Autodesk Inventor part; units mm, degrees
ref_plane "YZ Plane" through (0, 0, 0) normal (1, 0, 0) x (0, 1, 0)
ref_plane "XZ Plane" through (0, 0, 0) normal (0, 1, 0) x (-1, 0, 0)
ref_plane "XY Plane" through (0, 0, 0) normal (0, 0, 1) x (1, 0, 0)
sketch "Esboço1" plane through (0, 0, 0) normal (1, 0, 0) x (0, 1, 0)
  line L0 (-504, 129) -> (504, 129)
  line L1 (504, 129) -> (504, -129)
  line L2 (504, -129) -> (-504, -129)
  line L3 (-504, -129) -> (-504, 129)
  line L4 (-504, 129) -> (504, -129) construction
  line L5 (504, 129) -> (-504, -129) construction
  point P0 (0, 0)
  dimension "d0" = 1008
  dimension "d1" = 258
extrude "Extrusão1" add sketch "Esboço1" along normal mid plane 4
sketch "Esboço2" plane through (2, 0, 0) normal (1, 0, 0) x (0, 0, -1)
  line L0 (-133, 378) -> (-125, 378)
  line L1 (-125, 378) -> (-125, 126)
  line L2 (-125, 126) -> (-133, 126)
  line L3 (-133, 126) -> (-133, 378)
  line L4 (-129, 504) -> (-129, -504)
  line L5 (-133, 378) -> (-125, 126) construction
  line L6 (-125, 378) -> (-133, 126) construction
  line L7 (129, 504) -> (-129, 504)
  line L8 (-133, -126) -> (-125, -126)
  line L9 (-125, -126) -> (-125, -378)
  line L10 (-125, -378) -> (-133, -378)
  line L11 (-133, -378) -> (-133, -126)
  line L12 (-133, -126) -> (-125, -378) construction
  line L13 (-125, -126) -> (-133, -378) construction
  line L14 (-129, -504) -> (129, -504)
  line L15 (125, 378) -> (133, 378)
  line L16 (133, 378) -> (133, 126)
  line L17 (133, 126) -> (125, 126)
  line L18 (125, 126) -> (125, 378)
  line L19 (129, -504) -> (129, 504)
  line L20 (125, 378) -> (133, 126) construction
  line L21 (133, 378) -> (125, 126) construction
  line L22 (125, -126) -> (133, -126)
  line L23 (133, -126) -> (133, -378)
  line L24 (133, -378) -> (125, -378)
  line L25 (125, -378) -> (125, -126)
  line L26 (125, -126) -> (133, -378) construction
  line L27 (133, -126) -> (125, -378) construction
  point P0 (0, 0)
  point P1 (-129, 252)
  point P2 (-129, -252)
  point P3 (129, 252)
  point P4 (129, -252)
  dimension "d4" = 8
  dimension "d5" = 252
  dimension "d6" = 126
  dimension "d7" = 8
  dimension "d8" = 252
  dimension "d9" = 252
  dimension "d10" = 126
  dimension "d11" = 126
  dimension "d12" = 252
  dimension "d13" = 8
  dimension "d14" = 252
  dimension "d15" = 8
  dimension "d16" = 252
  dimension "d17" = 126
extrude "Extrusão2" cut sketch "Esboço2" along normal through all both and the other way through all contours L0 L4 L2 L3 | L0 L1 L2 L4 | L8 L9 L10 L4 | L4 L10 L11 L8 | L19 L17 L18 L15 | L15 L16 L17 L19 | L22 L23 L24 L19 | L19 L24 L25 L22
sketch "Esboço3" plane through (2, 0, 0) normal (1, 0, 0) x (0, 0, -1)
  line L0 (-41.5, 500) -> (41.5, 500)
  line L1 (41.5, 500) -> (41.5, 508)
  line L2 (41.5, 508) -> (-41.5, 508)
  line L3 (-41.5, 508) -> (-41.5, 500)
  line L4 (129, 504) -> (-129, 504)
  line L5 (-41.5, 500) -> (41.5, 508) construction
  line L6 (41.5, 500) -> (-41.5, 508) construction
  line L7 (-41.5, -500) -> (41.5, -500)
  line L8 (41.5, -500) -> (41.5, -508)
  line L9 (41.5, -508) -> (-41.5, -508)
  line L10 (-41.5, -508) -> (-41.5, -500)
  line L11 (-129, -504) -> (129, -504)
  line L12 (-41.5, -500) -> (41.5, -508) construction
  line L13 (41.5, -500) -> (-41.5, -508) construction
  point P0 (0, 0)
  point P1 (0, 504)
  point P2 (0, -504)
  dimension "d20" = 83
  dimension "d21" = 8
  dimension "d22" = 83
  dimension "d23" = 8
extrude "Extrusão3" cut sketch "Esboço3" along normal through all both and the other way through all
sketch "Esboço5" plane through (2, 0, 0) normal (1, 0, 0) x (0, 0, -1)
  line L0 (41.5, 500) -> (-41.5, 500)
  line L1 (0, 400) -> (-85, 400)
  line L2 (-125, 378) -> (-125, 126)
  line L3 (0, 400) -> (85, 400)
  line L4 (-85, 400) -> (-85, 166.6667)
  line L5 (-85, 166.6667) -> (85, 166.6667)
  line L6 (85, 166.6667) -> (85, 400)
  point P0 (0, 0)
  dimension "d39" = 85
  dimension "d40" = 85
  dimension "d41" = 233.3333
extrude "Extrusão5" cut sketch "Esboço5" against normal through all
pattern_linear "Padrão retangular2" count 3 spacing 283.3333 along (0, -1, 0) of "Extrusão5"
sketch "Esboço6" plane through (2, 0, 0) normal (1, 0, 0) x (0, 0, -1)
  line L0 (-85, -166.6667) -> (85, -166.6667)
  line L1 (85, -116.6667) -> (-85, -116.6667)
  line L2 (-85, -116.6667) -> (-35, -116.6667)
  line L3 (85, -116.6667) -> (35, -116.6667)
  line L4 (35, -116.6667) -> (-35, -116.6667)
  line L5 (-35, -129.1667) -> (35, -129.1667)
  line L6 (35, -129.1667) -> (35, -154.1667)
  line L7 (35, -154.1667) -> (-35, -154.1667)
  line L8 (-35, -129.1667) -> (-35, -154.1667)
  point P0 (0, 0)
  dimension "d47" = 50
  dimension "d48" = 50
  dimension "d49" = 50
  dimension "d50" = 12.5
  dimension "d51" = 25
extrude "Extrusão6" cut sketch "Esboço6" against normal through all
pattern_linear "Padrão retangular3" count 3 spacing 283.3333 along (0, 1, 0) of "Extrusão6"
sketch "Esboço7" plane through (2, 0, 0) normal (1, 0, 0) x (0, 0, -1)
  line L0 (-85, -400) -> (-85, -166.6667)
  line L1 (-125, -126) -> (-125, -378)
  line L2 (-85, 166.6667) -> (-85, 400)
  line L3 (-107.5, 280.8333) -> (-102.5, 280.8333)
  line L4 (-102.5, 280.8333) -> (-102.5, 285.8333)
  line L5 (-102.5, 285.8333) -> (-107.5, 285.8333)
  line L6 (-107.5, 285.8333) -> (-107.5, 280.8333)
  line L7 (-107.5, 280.8333) -> (-102.5, 285.8333) construction
  line L8 (-102.5, 280.8333) -> (-107.5, 285.8333) construction
  point P0 (0, 0)
  dimension "d60" = 5
  dimension "d61" = 5
extrude "Extrusão7" cut sketch "Esboço7" against normal through all
pattern_linear "Padrão retangular4" count 3 spacing 283.3333 along (0, -1, 0) of "Extrusão7"
properties part number "PAREDE FRONTAL"
Check sheet for the modelled part. Datum: model origin and axes. Units: mm. Round coordinates to 2 decimals unless told otherwise and drop trailing zeros. Write each loop counter-clockwise with the first axis right and the second up, starting at its lowest first coordinate (ties: lowest second). Pieces come first, ordered by that corner, then holes. Notation, with made-up numbers: (-10.75, 75) -> (8.25, 75) arc R37 cw to (8.25, 113) -> close; hole circle Ø4 at (-36, -33). An arc over 180 degrees is marked (long way). One line per question, with ' | ' between items. Start each with the question number.
1. Sectioned sample at D-D, the plane y = -352. Record the cut outline in (x, z).
2. Sectioned sample at C-C, the plane z = 4. Record the cut outline in (x, y), then the cut area to 3 significant figures.
3. Sectioned sample at A-A, the plane y = -68.5. Record the cut outline in (x, z).
4. Sectioned sample at B-B, the plane z = -63. Record the cut outline in (x, y).
5. Depth check by flat-ended pin: pin 1 (1.2 mm diameter, centred on x = 0.5, y = 302.5, fed in from +Z); pin 2 (1.2 mm diameter, centred on x = 0, z = 0.5, fed in from +Y). Enter the tip coordinate at first touch or a pass-through.
6. Scan lines: line 1 along Y through (x, z) = (0.55, 45.5); line 2 along Z through (x, y) = (1.7, -130.5); line 3 along Z through (x, y) = (0.3, -192.5). Record each from-to range of solid material in increasing order. Write a range as from..to.
Taken from the geometry:
1) outline: (-2, -125) -> (2, -125) -> (2, -85) -> (-2, -85) -> close; (-2, 85) -> (2, 85) -> (2, 125) -> (-2, 125) -> close
2) outline: (-2, -500) -> (2, -500) -> (2, -400) -> (-2, -400) -> close; (-2, -166.67) -> (2, -166.67) -> (2, -154.17) -> (-2, -154.17) -> close; (-2, -129.17) -> (2, -129.17) -> (2, -116.67) -> (-2, -116.67) -> close; (-2, 116.67) -> (2, 116.67) -> (2, 129.17) -> (-2, 129.17) -> close; (-2, 154.17) -> (2, 154.17) -> (2, 166.67) -> (-2, 166.67) -> close; (-2, 400) -> (2, 400) -> (2, 412.5) -> (-2, 412.5) -> close; (-2, 437.5) -> (2, 437.5) -> (2, 500) -> (-2, 500) -> close | area: 900 mm^2
3) outline: (-2, -129) -> (2, -129) -> (2, -85) -> (-2, -85) -> close; (-2, 85) -> (2, 85) -> (2, 129) -> (-2, 129) -> close
4) outline: (-2, -504) -> (2, -504) -> (2, -400) -> (-2, -400) -> close; (-2, -166.67) -> (2, -166.67) -> (2, -116.67) -> (-2, -116.67) -> close; (-2, 116.67) -> (2, 116.67) -> (2, 166.67) -> (-2, 166.67) -> close; (-2, 400) -> (2, 400) -> (2, 504) -> (-2, 504) -> close
5) pin 1: stops at z = 125 | pin 2: stops at y = 500
6) line 1: y = -504..-400, -166.67..-116.67, 116.67..166.67, 400..504 | line 2: z = -125..-35, 35..125 | line 3: z = -125..-85, 85..125
